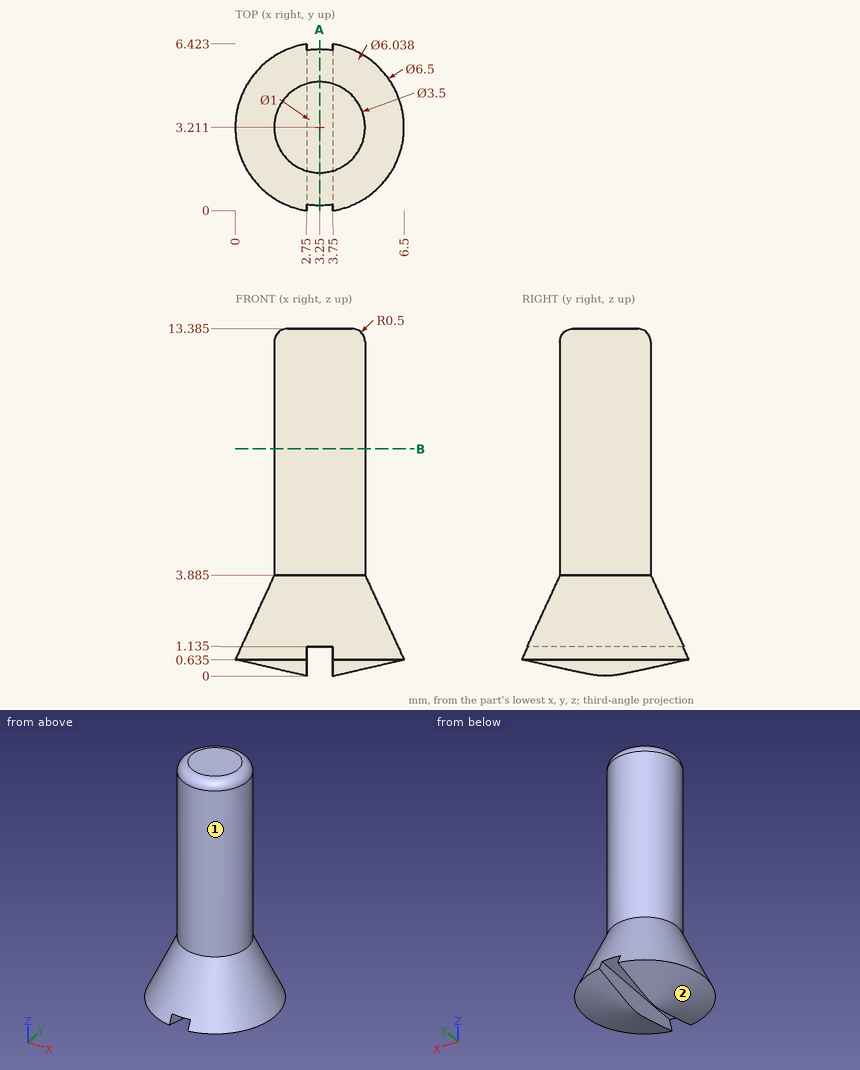
Verification items for this drawing (mm, ordinates from the low corner). A direction names the side the tool comes from. Coordinates: 2 decimals unless noted, no trailing zeros. Write each loop counter-clockwise with the first axis right and the second up, starting at its lowest first coordinate (ties: lowest second). Pieces come first, ordered by that corner, then holes. Notation, with made-up numbers: (20.25, 32.5) -> (47.25, 32.5) arc R32 ccw to (47.25, 69.5) -> close; hole circle Ø4 at (76.25, 81.5). An arc over 180 degrees is marked (long way). Use CSV: the item, a comma, the result in double quotes. Start each with the question number.
Item 1: Depth check by flat-ended pin: pin 1 Ø3 at (x, y) = (2, 4.5) entering from -Z; pin 2 Ø2 at (x, z) = (4.5, 7.5) entering from +Y; pin 3 Ø1.5 at (y, z) = (2.5, 10.5) entering from +X; pin 4 Ø1.5 at (x, z) = (3.5, 5.5) entering from -Y. Enter the tip coordinate at first touch or a pass-through.
Item 2: Cross-section at A-A, the plane x = 3.25. Record the cut outline in (y, z) (1 decimal).
Item 3: Thickness scan on line 1 (X direction, y = 3.25, z = 11); line 2 (Z direction, x = 3.5, y = 3.75) (1 decimal); line 3 (X direction, y = 2.5, z = 9). Record the ranges inside material, lowest first.
Item 4: Cross-section at B-B, the plane z = 8.75. Record the cut outline in (x, y).
Item 5: Set-up check for the marked faces 1 and 2: record each of +Z, -Z, +X, -X, +Y, -Y from which the full face is reachable in a straight line by a thin tool's end or side.
Answers:
1,pin 1,"z = 0"
1,pin 2,"y = 4.94"
1,pin 3,"x = 5"
1,pin 4,"y = 1.46"
2,outline,"(0.2, 1.1) -> (6.2, 1.1) -> (5, 3.9) -> (5, 12.9) arc R0.5 ccw to (4.5, 13.4) -> (2, 13.4) arc R0.5 ccw to (1.5, 12.9) -> (1.5, 3.9) -> close"
3,line 1,"1.5 to 5"
3,line 2,"1.1 to 13.4"
3,line 3,"1.65 to 4.85"
4,outline,"circle Ø3.5 at (3.25, 3.21)"
5,face 1,"+Z"
5,face 2,"-Z, -X"
